Autodesk Inventor part; units mm, degrees
ref_plane "Начальная плоскость" through (0, 0, 58.9006) normal (0, 0, 1) x (1, 0, 0)
ref_plane "Конечная плоскость" through (0, 0, 458.193) normal (0, 0, 1) x (1, 0, 0)
ref_plane "РабПлоскость8" through (36, -195.6097, 277.8202) normal (0, -0.6924, -0.7215) x (1, 0, 0)
ref_plane "Начальная плоскость" through (0, 0, 58.9006) normal (0, 0, 1) x (1, 0, 0)
ref_plane "Конечная плоскость" through (0, 0, 458.193) normal (0, 0, 1) x (1, 0, 0)
sketch "Эскиз" plane through (0, 0, 0) normal (0, 0, 1) x (1, 0, 0)
  line L0 (36, -32.5) -> (0, -32.5)
  line L1 (36, -32.5) -> (36, -28.696)
  line L2 (33.6994, -26.2039) -> (9.9215, -24.3017)
  line L3 (4.4, -18.3208) -> (4.4, 18.3208)
  line L4 (33.6994, 26.2039) -> (9.9215, 24.3017)
  line L5 (36, 28.696) -> (36, 32.5)
  line L6 (0, 32.5) -> (36, 32.5)
  line L7 (0, -32.5) -> (0, 32.5)
  arc A0 (4.4, -18.3208) -> (9.9215, -24.3017) centre (10.4, -18.3208) ccw
  arc A1 (9.9215, 24.3017) -> (4.4, 18.3208) centre (10.4, 18.3208) ccw
  arc A2 (36, -28.696) -> (33.6994, -26.2039) centre (33.5, -28.696) ccw
  arc A3 (33.6994, 26.2039) -> (36, 28.696) centre (33.5, 28.696) ccw
  line L8 (0, 45.5) -> (0, -45.5) construction
  line L9 (-7.2974, 0) -> (43.7847, 0) construction
  point P0 (36, -26.388)
  point P1 (4.4, -23.86)
  point P2 (4.4, 23.86)
  point P3 (36, 26.388)
  dimension "d3" = 36
  dimension "d5" = 4.4
  dimension "d7" = 65
  dimension "d9" = 8.64
  dimension "d11" = 8.64
  dimension "d13" = 6.112
  dimension "d15" = 6.112
  dimension "d22" = 6
  dimension "d23" = 2.5
  dimension "d24" = 32.5
  dimension "d25" = 0
extrude "Тело" add sketch "Эскиз" along normal up to surface (399.2924 mm away) from surface at 58.9006
sketch "Sketch3" plane through (0, 0, 0) normal (0, 0, 1) x (1, 0, 0)
  line L0 (0, 0) -> (10, 0)
ref_plane "Work Plane7" through (0, 0, 0) normal (0, -1, 0) x (1, 0, 0)
sketch "Sketch4" plane through (0, 0, 0) normal (0, -1, 0) x (1, 0, 0)
  line L0 (-2, 58.9006) -> (12, 58.9006)
  line L1 (-2, 458.193) -> (12, 458.193)
  dimension "d29" = 399.2924
ref_plane "РабПлоскость8" through (36, -195.6097, 277.8202) normal (0, -0.6924, -0.7215) x (1, 0, 0)
split "Разделение1" plane through (36, -195.6097, 277.8202) removes the side toward (0, -0.6924, -0.7215)
ref_plane "РабПлоскость9" through (0, -22.5038, 458.193) normal (0, 0.6924, 0.7215) x (1, 0, 0)
split "Разделение2" plane through (0, -22.5038, 458.193) removes the side toward (0, 0.6924, 0.7215)
ref_plane "РабПлоскость10" through (-29, 195.6464, 685.5009) normal (0, -0.7215, 0.6924) x (1, 0, 0)
split "Разделение3" plane through (-29, 195.6464, 685.5009) removes the side toward (0, -0.7215, 0.6924)
equation "\"d3\" = b"
equation "\"d7\" = ParH"
equation "\"d22\" = R"
equation "\"d23\" = R1"
equation "\"d24\" = 0.5 * d7"
equation "\"d16\" = G_L"
equation "\"R1\" = 2.5"
equation "\"R\" = 6"
equation "\"t1\" = 4.4"
equation "\"t2\" = 7.2"
equation "\"ParH\" = 65"
equation "\"b\" = 36"
equation "\"msp_x1\" = 0.04 * b"
equation "\"msp_x2\" = -0.08 * t1 + 0.04 * b"
equation "\"G_L\" = d29"
equation "\"ex\" = 0"
equation "\"G_OFFSET_START\" = -58.90056"
equation "\"G_OFFSET_END\" = -23.44846"
equation "\"d26\" = -G_OFFSET_START"
equation "\"d27\" = G_OFFSET_END + B_L"
equation "\"B_L\" = 481.64146"
properties part number "Швеллер 6.5U-399,29 ГОСТ 8240-97" material "Сталь, мягкая"
The model under review builds one solid part; all positions refer to its coordinate system, in mm. A direction names the side the tool comes from. Give positions to 0.01 mm unless a question says otherwise; leave off trailing zeros. Write each loop counter-clockwise with the first axis right and the second up, starting at its lowest first coordinate (ties: lowest second). Pieces come first, ordered by that corner, then holes. Notation, with made-up numbers: (74.5, 16) - (121.5, 16) arc R26 cw to (121.5, 38) - close; hole circle Ø1 at (50.25, -1). An arc over 180 degrees is marked (long way). Answer in a Markdown table with one row per item. Add a question column.
1. Wall thickness on line 1 along Y through (x, z) = (10, 153); line 2 along Y through (x, z) = (10.5, 439.5); line 3 along X through (y, z) = (15, 100): over which ranges is each line inside the solid? List them lowest first. Write a range as [from, to].
2. We need section A-A on x = 20. Write out the cut boundary in (y, z).
3. Insertion check: P1, Ø6, axis at y = -13, z = 206.5, coming from the -X side; P2, Ø1, axis at y = -0.5, z = 316.5, coming from the +X side; P3, Ø10, axis at x = 12.5, y = 0.5, coming from the -Z side. Each pin has a flat end and moves straight along its axis. Give the tip position at first contact, or say it passes through.
4. Draft analysis for pull direction Y (two halves, no side actions). For faces 3 (the flat face through (18, 32.5, 230)), 4 (the flat face through (21.977, 25.266, 236.676)), 5 (the flat face through (0, 0, 256)), state which applies: +Y half, -Y half, draft (parallel to the pull), parting line (faces both ways), or undercut.
5. We need section C-C on y = 7.5. Write out the cut boundary in (x, z).
6. We need section B-B on z = 369.5. Write out the cut boundary in (x, y).
7. Tool access review of faces 1 (the flat face through (21.977, -25.266, 282.465)), 2 (the flat face through (18, -32.5, 282)): name each direction out of +Z, -Z, +X, -X, +Y, -Y from which nothing blocks a thin tool from reaching the whole face with its end or side.
Ans:
| question | item | result |
|---|---|---|
| 1 | line 1 | y = [-32.5, -24.31], [24.31, 32.5] |
| 1 | line 2 | y = [-32.5, -24.35] |
| 1 | line 3 | x = [0, 4.4] |
| 2 | outline | (-32.5, 121.29) - (-25.11, 114.2) - (-25.11, 455.47) - (-32.5, 447.77) - close; (25.11, 66) - (32.5, 58.91) - (32.5, 405.41) - (25.11, 412.5) - close |
| 3 | P1 | stops at x = 0 |
| 3 | P2 | stops at x = 4.4 |
| 3 | P3 | passes through |
| 4 | face 3 | +Y half |
| 4 | face 4 | undercut |
| 4 | face 5 | draft |
| 5 | outline | (0, 82.9) - (4.4, 82.9) - (4.4, 429.4) - (0, 429.4) - close |
| 6 | outline | (0, -32.5) - (36, -32.5) - (36, -28.7) arc R2.5 ccw to (33.7, -26.2) - (9.92, -24.3) arc R6 cw to (4.4, -18.32) - (4.4, 18.32) arc R6 cw to (9.92, 24.3) - (33.7, 26.2) arc R2.5 ccw to (36, 28.7) - (36, 32.5) - (0, 32.5) - close |
| 7 | face 1 | +Z, -Z, +X |
| 7 | face 2 | +Z, -Z, +X, -X, -Y |
